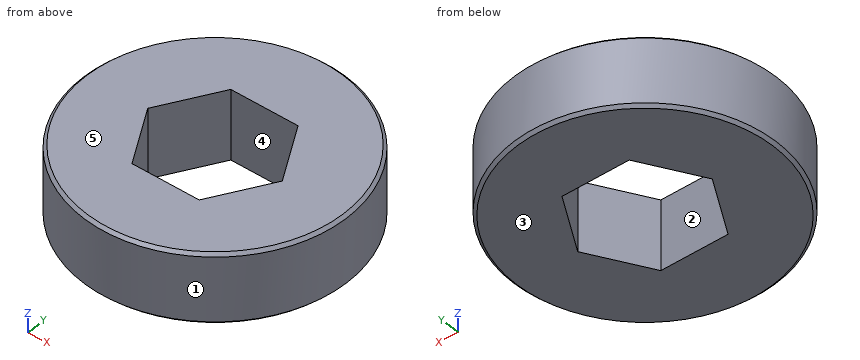
```python
from build123d import *

# Parameters (mm, degrees)
F0_R     = 14.3002
F1_DEPTH = 3.81
F2_SIZE  = 0.3175


with BuildPart() as f1:
    # F0 (on Top) → F1 (new body, symmetric)
    with BuildSketch(Plane.XY):
        Circle(F0_R)
        Polygon((-3.6661742094, 6.35), (3.6661742094, 6.35), (7.3323484187, 0), (3.6661742094, -6.35), (-3.6661742094, -6.35), (-7.3323484187, 0), align=None, mode=Mode.SUBTRACT)
    extrude(amount=F1_DEPTH, both=True)

    # F2
    f2_edges = [f1.edges().sort_by_distance(p)[0] for p in [
        (-14.3002, 0, 3.81),
        (-14.3002, 0, -3.81),
    ]]
    chamfer(f2_edges, length=F2_SIZE)


solid = f1.part
```
For this review, take the finished solid that the model builds, in its own axes (mm). Face numbers are marked on the shaded views. A direction names the side the tool comes from. Coordinates: 2 decimals unless noted, no trailing zeros. Loops run counter-clockwise (first coordinate to the right, second up) from the corner with the lowest first, then second, coordinate; pieces in that order, holes last.
1. Mouldability with a two-part tool opening along X and no side actions: class the marked faces 1, 2 and 3 as +X half, -X half, draft (parallel to the pull), parting line (faces both ways), or undercut.
2. For line 1 (X direction, y = 1.25, z = 1.5); line 2 (X direction, y = 1.5, z = -0.75); line 3 (Y direction, x = -7, z = 0.25), list the stretches that pass through material, from the lowest coordinate up.
3. Add section B-B, the plane z = 3. Give the boundary of the cut face in (x, y), then the cut area to 3 significant figures.
4. Insertion check: P1, Ø3, axis at y = -9.5, z = 1, coming from the +X side; P2, Ø4, axis at x = -7.5, z = 1.5, coming from the +Y side; P3, Ø1.5, axis at x = 6.5, z = 2.5, coming from the -Y side. Each pin has a flat end and moves straight along its axis. Give the tip position at first contact, or say it passes through.
5. Add section A-A, the plane x = 0. Give the boundary of the cut face in (y, z).
6. For the marked faces 4 and 5, list the 3-axis set-ups (+Z, -Z, +X, -X, +Y, -Y) from which the entire face can be reached by the end or side of a thin tool; tool diameter is ignored.
Result:
1. face 1: parting line
1. face 2: undercut
1. face 3: draft
2. line 1: x = -14.25 to -6.61, 6.61 to 14.25
2. line 2: x = -14.22 to -6.47, 6.47 to 14.22
2. line 3: y = -12.47 to -0.58, 0.58 to 12.47
3. outline: circle Ø28.6 at (0, 0); hole (-7.33, 0) - (-3.67, -6.35) - (3.67, -6.35) - (7.33, 0) - (3.67, 6.35) - (-3.67, 6.35) - close
3. area: 503 mm2
4. P1: stops at x = 11.85
4. P2: stops at y = 13.2
4. P3: stops at y = -13.09
5. outline: (-14.3, -3.49) - (-13.98, -3.81) - (-6.35, -3.81) - (-6.35, 3.81) - (-13.98, 3.81) - (-14.3, 3.49) - close; (6.35, -3.81) - (13.98, -3.81) - (14.3, -3.49) - (14.3, 3.49) - (13.98, 3.81) - (6.35, 3.81) - close
6. face 4: +Z, -Z
6. face 5: +Z, +X, -X, +Y, -Y
